Can you work these out from the drawing? Everything is in mm from the part's minimum corner. A direction names the side the tool comes from. Round coordinates to 2 decimals unless told otherwise and drop trailing zeros. Write each loop counter-clockwise with the first axis right and the second up, starting at its lowest first coordinate (ties: lowest second). Pieces come first, ordered by that corner, then holes. Notation, with made-up numbers: (-10, 66) -> (17, 66) arc R11 cw to (17, 77) -> close; hole circle Ø8 at (-17, -13.5). An arc over 180 degrees is marked (long way). One line per question, with ' | ' between items. Start each with the question number.
1. For the marked faces 5, 6 and 7, which set-ups out of +Z, -Z, +X, -X, +Y, -Y let a thin tool reach every point of the face, with its end or its side?
2. Imagine slicing it at B-B, the plane x = 60.5. List the corners of the cut face in (y, z) for me.
3. Imagine slicing it at A-A, the plane z = 15.5. List the corners of the cut face in (x, y) for me, and give its area (3 significant figures).
4. Imagine slicing it at D-D, the plane y = 52. List the corners of the cut face in (x, z) for me, and give its area (3 significant figures).
5. If I drill on line 1 along Y through (x, z) = (80, 30); line 2 along X through (y, z) = (60.5, 5.5); line 3 along Y through (x, z) = (55.5, 3.5), over which ranges is the centre line in solid material (lowest first)? Write a range as [from, to].
6. For pin 1 Ø1 at (y, z) = (23, 15) entering from +X; pin 2 Ø7.5 at (x, y) = (44.5, 25) entering from -Z; pin 3 Ø7.5 at (x, y) = (45.5, 20) entering from +Z; pin 4 Ø2.5 at (y, z) = (67, 17) entering from -X, each with a flat end and sliding along its axis, tell me the tip position at first contact or that it passes through.
7. Imagine slicing it at C-C, the plane y = 6.35. List the corners of the cut face in (x, z) for me (1 decimal).
8. Thinking about a two-plate mould opening in X: for the marked faces 1, 2, 3 and 4, which applies, released by +X, released by -X, zero draft, split by the parting line, or undercut?
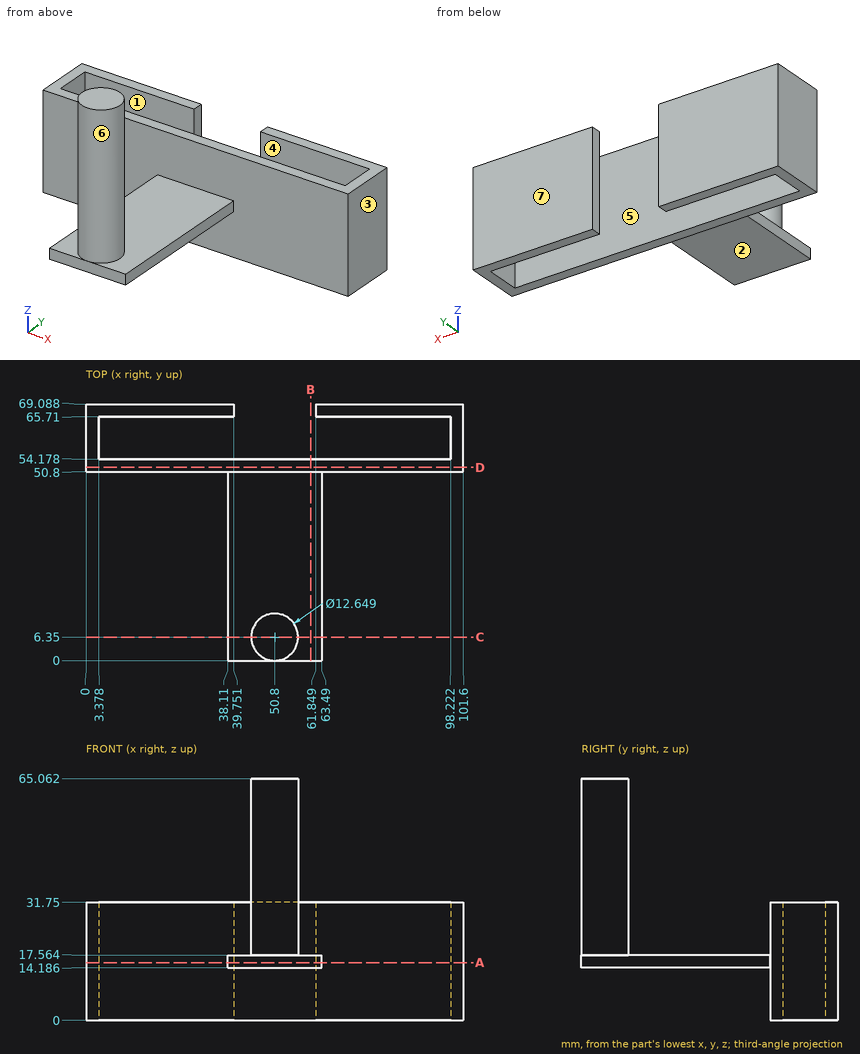
Geometry results:
1) face 5: +Z, -Z | face 6: +Z | face 7: +Z, -Z, +X, -X, +Y
2) outline: (0, 14.19) -> (50.8, 14.19) -> (50.8, 0) -> (54.18, 0) -> (54.18, 31.75) -> (50.8, 31.75) -> (50.8, 17.56) -> (0, 17.56) -> close
3) outline: (0, 50.8) -> (38.11, 50.8) -> (38.11, 0) -> (63.49, 0) -> (63.49, 50.8) -> (101.6, 50.8) -> (101.6, 69.09) -> (61.85, 69.09) -> (61.85, 65.71) -> (98.22, 65.71) -> (98.22, 54.18) -> (3.38, 54.18) -> (3.38, 65.71) -> (39.75, 65.71) -> (39.75, 69.09) -> (0, 69.09) -> close | area: 1,980 mm2
4) outline: (0, 0) -> (101.6, 0) -> (101.6, 31.75) -> (0, 31.75) -> close | area: 3,230 mm2
5) line 1: y = [50.8, 54.18], [65.71, 69.09] | line 2: x = [0, 3.38], [98.22, 101.6] | line 3: y = [50.8, 54.18]
6) pin 1: stops at x = 63.49 | pin 2: stops at z = 14.19 | pin 3: stops at z = 17.56 | pin 4: stops at x = 0
7) outline: (38.1, 14.2) -> (63.5, 14.2) -> (63.5, 17.6) -> (57.1, 17.6) -> (57.1, 65.1) -> (44.5, 65.1) -> (44.5, 17.6) -> (38.1, 17.6) -> close
8) face 1: undercut | face 2: zero draft | face 3: released by +X | face 4: undercut
